Job drawing, mm, ordinate dimensions from the low corner. One solid piece. A direction names the side the tool comes from. Coordinates: 2 decimals unless noted, no trailing zeros. Loops run counter-clockwise (first coordinate to the right, second up) from the corner with the lowest first, then second, coordinate; pieces in that order, holes last. Notation, with made-up numbers: M 33,14 L 41,14 A27 ccw 41,51 Z; hole C 42.5,84 d3. An arc over 180 degrees is marked long. Answer as a JSON object with one key per item and string values. Group by question number.
1. 3-axis set-ups, long thin cutter, end or side, ignore diameter. For the marked faces 5, 6 and 7: which of +Z, -Z, +X, -X, +Y, -Y reach the whole face in a straight line?
2. Saw through at A-A on z = 6.5. Write the cut outline in (x, y), then the cut area to 3 significant figures.
3. Mould opens along Z. For the marked faces 1, 2, 3 and 4 say: released by +Z, released by -Z, zero draft, split by the parting line, or undercut.
4. Drill centre lines: L1, parallel to X at y = 17.5, z = 16.5; L2, parallel to Z at x = 27, y = 6.25; L3, parallel to Y at x = 17.5, z = 12.5. Where is each one in solid material? Low to high.
5. Drop flat-ended pins along their axis: pin 1 Ø7 at (x, y) = (28.5, 6) entering from +Z; pin 2 Ø1.1 at (x, z) = (32.5, 10.5) entering from -Y; pin 3 Ø4 at (x, z) = (16.5, 6.5) entering from +Y; pin 4 Ø3 at (x, y) = (31.5, 12.5) entering from -Z. Give the stop position or say it passes through.
6. Saw through at B-B on y = 15.75. Write the cut outline in (x, z).
7. Saw through at D-D on z = 12. Write the cut outline in (x, y).
8. Saw through at C-C on y = 2. Write the cut outline in (x, z).
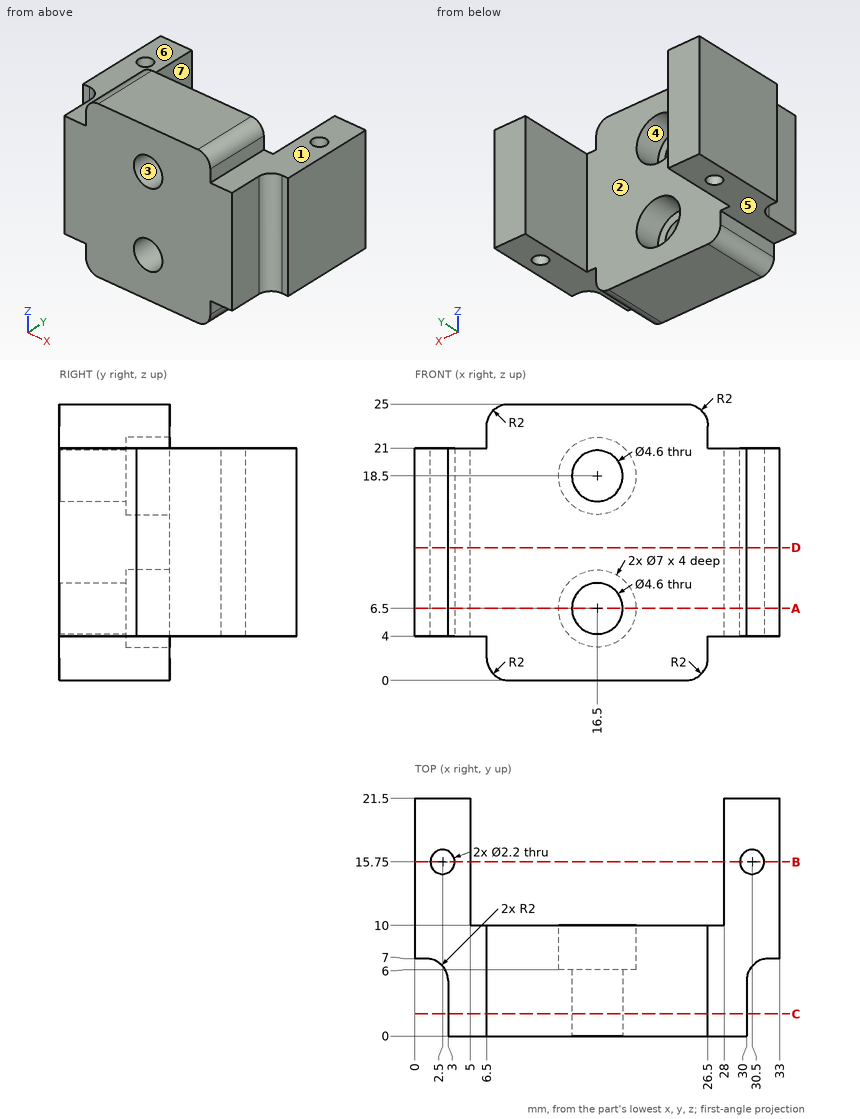
Outcome:
{
 "1": {"face 5": "-Z, -X, +Y, -Y", "face 6": "+Z, -X, +Y, -Y", "face 7": "+Z, -Z, +Y"},
 "2": {"outline": "M 0,7 L 1,7 A2 cw 3,5 L 3,0 L 14.2,0 L 14.2,6 L 13,6 L 13,10 L 5,10 L 5,21.5 L 0,21.5 Z; M 18.8,0 L 30,0 L 30,5 A2 cw 32,7 L 33,7 L 33,21.5 L 28,21.5 L 28,10 L 20,10 L 20,6 L 18.8,6 Z; hole C 2.5,15.75 d2.2; hole C 30.5,15.75 d2.2", "area": "342 mm²"},
 "3": {"face 1": "released by +Z", "face 2": "zero draft", "face 3": "undercut", "face 4": "undercut"},
 "4": {"L1": "x = 0 to 5, 28 to 33", "L2": "z = 4 to 21", "L3": "y = 0 to 10"},
 "5": {"pin 1": "stops at z = 24.94", "pin 2": "stops at y = 7", "pin 3": "passes through", "pin 4": "stops at z = 4"},
 "6": {"outline": "M 0,4 L 1.4,4 L 1.4,21 L 0,21 Z; M 3.6,4 L 5,4 L 5,21 L 3.6,21 Z; M 28,4 L 29.4,4 L 29.4,21 L 28,21 Z; M 31.6,4 L 33,4 L 33,21 L 31.6,21 Z"},
 "7": {"outline": "M 0,7 L 1,7 A2 cw 3,5 L 3,0 L 30,0 L 30,5 A2 cw 32,7 L 33,7 L 33,21.5 L 28,21.5 L 28,10 L 5,10 L 5,21.5 L 0,21.5 Z; hole C 2.5,15.75 d2.2; hole C 30.5,15.75 d2.2"},
 "8": {"outline": "M 3,4 L 6.5,4 L 6.5,2 A2 ccw 8.5,0 L 24.5,0 A2 ccw 26.5,2 L 26.5,4 L 30,4 L 30,21 L 26.5,21 L 26.5,23 A2 ccw 24.5,25 L 8.5,25 A2 ccw 6.5,23 L 6.5,21 L 3,21 Z; hole C 16.5,6.5 d4.6; hole C 16.5,18.5 d4.6"}
}
